Input: part model. Units: mm. Frame: model coordinates. A direction names the side the tool comes from. Give positions to 0.01 mm unless a question says otherwise; leave off trailing zeros. Write each loop counter-clockwise with the first axis right and the second up, starting at its lowest first coordinate (ties: lowest second). Pieces come first, ordered by that corner, then holes. Notation, with made-up numbers: (57, -14.75) - (78, -14.75) arc R16 cw to (78, 11.25) - close; hole circle Ø11 at (-6.5, -27.5). An arc over 180 degrees is marked (long way). Answer as a JSON object with one key per item and string values. Group by question number.
from build123d import *

# Parameters (mm, degrees)
SKETCH1_R           = 7
SKETCH1_R_2         = 2.5
BOSS_EXTRUDE1_DEPTH = 5
SKETCH2_R           = 3.024719142
SKETCH2_R_2         = 2.760237687
CUT_EXTRUDE1_DEPTH  = 0.5
SKETCH3_R           = 6.500951531
SKETCH3_R_2         = 6.143653391
CUT_EXTRUDE2_DEPTH  = 0.5
SKETCH4_R           = 6.653685529
SKETCH4_R_2         = 6.402971613
SKETCH4_R_3         = 3.211895498
SKETCH4_R_4         = 2.91485273
CUT_EXTRUDE3_DEPTH  = 0.5


with BuildPart() as part:
    # Sketch1 → Boss-Extrude1 (new body)
    with BuildSketch(Plane(origin=(0, 0, 0), x_dir=(1, 0, 0), z_dir=(0, 1, 0))):
        with Locations(Location((0, 0, 0), (0, 0, 270))):
            Circle(SKETCH1_R)
        with Locations(Location((0, 0, 0), (0, 0, 270))):
            Circle(SKETCH1_R_2, mode=Mode.SUBTRACT)
    extrude(amount=BOSS_EXTRUDE1_DEPTH)

    # Sketch2 → Cut-Extrude1 (cut)
    with BuildSketch(Plane(origin=(0, 5, 0), x_dir=(1, 0, 0), z_dir=(0, 1, 0))):
        with Locations(Location((0, 0, 0), (0, 0, 270))):
            Circle(SKETCH2_R)
        with Locations(Location((0, 0, 0), (0, 0, 270))):
            Circle(SKETCH2_R_2, mode=Mode.SUBTRACT)
    extrude(amount=-CUT_EXTRUDE1_DEPTH, mode=Mode.SUBTRACT)

    # Sketch3 → Cut-Extrude2 (cut)
    with BuildSketch(Plane(origin=(0, 5, 0), x_dir=(1, 0, 0), z_dir=(0, 1, 0))):
        with Locations(Location((0, 0, 0), (0, 0, 270))):
            Circle(SKETCH3_R)
        with Locations(Location((0, 0, 0), (0, 0, 270))):
            Circle(SKETCH3_R_2, mode=Mode.SUBTRACT)
    extrude(amount=-CUT_EXTRUDE2_DEPTH, mode=Mode.SUBTRACT)

    # Sketch4 → Cut-Extrude3 (cut)
    with BuildSketch(Plane.XZ):
        with Locations(Location((0, 0, 0), (0, 0, 270))):
            Circle(SKETCH4_R)
        with Locations(Location((0, 0, 0), (0, 0, 270))):
            Circle(SKETCH4_R_2, mode=Mode.SUBTRACT)
        with Locations(Location((0, 0, 0), (0, 0, 270))):
            Circle(SKETCH4_R_3)
        with Locations(Location((0, 0, 0), (0, 0, 270))):
            Circle(SKETCH4_R_4, mode=Mode.SUBTRACT)
    extrude(amount=-CUT_EXTRUDE3_DEPTH, mode=Mode.SUBTRACT)


solid = part.part
1) Cut plane A-A on x = 5.25. Return the cut outline in (y, z), and give its area (3 significant figures).
2) Mould query, pull axis Z, two halves, no side actions, for faces 4 (the face through (-6.346, 4.754, -1.409)), 5 (the face through (-2.44, 2.46, -0.54)), 6 (the face through (-6.834, 2.465, -1.517)), 7 (the face through (2, 0, -3)). Classes: +Z half, -Z half, draft (parallel to the pull), parting line (faces both ways), or undercut.
3) Reachability of faces 1 (the face through (0.13, 0.25, 2.91)), 2 (the face through (-1.68, 4.75, -2.19)), 3 (the face through (1.5, 5, -2.8)) from +Z, -Z, +X, -X, +Y, -Y: full face, straight path, thin tool, end or side. Return the list, or none.
4) Line query: line 1 along X through (y, z) = (0.35, 0); line 2 along X through (y, z) = (4.75, 0); line 3 along Z through (x, y) = (-4.5, 0.4) (3 decimals). Output: solid intervals per line, ascending. Write a range as from..to.
5) Cut plane B-B on y = 4.1. Return the cut outline in (x, z).
6) Pin query (flat end, axial travel): P1, Ø4, axis at x = 0, z = 0, coming from the +Y side; P2, Ø3, axis at x = 1, z = -0.5, coming from the -Y side; P3, Ø3, axis at x = -3, y = 1, coming from the -Z side. Return the tip coordinate at first contact, or that it passes through.
7) Cut plane C-C on z = 3.5. Return the cut outline in (x, y).
Filled in:
{
 "1": {"outline": "(0, -4.63) - (5, -4.63) - (5, -3.83) - (4.5, -3.83) - (4.5, -3.19) - (5, -3.19) - (5, 3.19) - (4.5, 3.19) - (4.5, 3.83) - (5, 3.83) - (5, 4.63) - (0, 4.63) - (0, 4.09) - (0.5, 4.09) - (0.5, 3.67) - (0, 3.67) - (0, -3.67) - (0.5, -3.67) - (0.5, -4.09) - (0, -4.09) - close", "area": "45.2 mm²"},
 "2": {"face 4": "undercut", "face 5": "undercut", "face 6": "parting line", "face 7": "draft"},
 "3": {"face 1": "-Y", "face 2": "+Y", "face 3": "+Z, -Z, +X, -X, +Y"},
 "4": {"line 1": "x = -7..-6.65, -6.4..-3.21, -2.91..-2.5, 2.5..2.91, 3.21..6.4, 6.65..7", "line 2": "x = -7..-6.5, -6.14..-3.02, -2.76..-2.5, 2.5..2.76, 3.02..6.14, 6.5..7", "line 3": "z = -5.362..-4.901, -4.555..4.555, 4.901..5.362"},
 "5": {"outline": "circle Ø14 at (0, 0); hole circle Ø5 at (0, 0)"},
 "6": {"P1": "passes through", "P2": "stops at y = 0", "P3": "stops at z = -6.84"},
 "7": {"outline": "(-6.06, 0) - (-5.66, 0) - (-5.66, 0.5) - (-5.36, 0.5) - (-5.36, 0) - (5.36, 0) - (5.36, 0.5) - (5.66, 0.5) - (5.66, 0) - (6.06, 0) - (6.06, 5) - (5.48, 5) - (5.48, 4.5) - (5.05, 4.5) - (5.05, 5) - (-5.05, 5) - (-5.05, 4.5) - (-5.48, 4.5) - (-5.48, 5) - (-6.06, 5) - close"}
}
